For this review, take the finished solid that the model builds, in its own axes (mm). Give positions to 0.01 mm unless a question says otherwise; leave off trailing zeros. Loops run counter-clockwise (first coordinate to the right, second up) from the corner with the lowest first, then second, coordinate; pieces in that order, holes last. Notation, with made-up numbers: (79.25, -21.75) -> (120.25, -21.75) arc R16 cw to (120.25, -15.75) -> close; hole circle Ø5 at (-39.5, 83). An arc over 180 degrees is marked (long way). Write each question's results on one line, items separated by ' | '. Start each with the question number.
```python
from build123d import *

# Parameters (mm, degrees)
SKETCH1_R           = 12.7
BOSS_EXTRUDE1_DEPTH = 58.7248
CHAMFER3_SIZE       = 6.35
CHAMFER3_SIZE2      = 23.698522628
CHAMFER4_SIZE       = 6.35
CHAMFER4_SIZE2      = 23.698522628


with BuildPart() as part:
    # Sketch1 → Boss-Extrude1 (new body)
    with BuildSketch(Plane.XY):
        Circle(SKETCH1_R)
    extrude(amount=-BOSS_EXTRUDE1_DEPTH)

    # Chamfer3
    chamfer3_edges = [part.edges().sort_by_distance(p)[0] for p in [
        (-12.7, 0, -58.7248),
    ]]
    chamfer3_side = [part.faces().sort_by_distance(p)[0] for p in [
        (0, 0, -58.7248),
    ]]
    chamfer(chamfer3_edges, length=CHAMFER3_SIZE, length2=CHAMFER3_SIZE2, reference=chamfer3_side[0])

    # Chamfer4
    chamfer4_edges = [part.edges().sort_by_distance(p)[0] for p in [
        (-12.7, 0, 0),
    ]]
    chamfer4_side = [part.faces().sort_by_distance(p)[0] for p in [
        (0, 0, 0),
    ]]
    chamfer(chamfer4_edges, length=CHAMFER4_SIZE, length2=CHAMFER4_SIZE2, reference=chamfer4_side[0])


solid = part.part
```
1. Wall thickness on L1, parallel to Y at x = 5.75, z = -13; L2, parallel to Y at x = 7.5, z = -36.5; L3, parallel to X at y = -8.75, z = -17: over which ranges is each line inside the solid? List them lowest first.
2. We need section A-A (x = 0). Write out the cut boundary in (y, z).
3. We need section C-C (z = -55). Write out the cut boundary in (x, y).
4. For pin 1 Ø2 at (y, z) = (-2.5, -39) entering from +X; pin 2 Ø2 at (y, z) = (-8, -31) entering from +X; pin 3 Ø8 at (x, z) = (8.5, -27.5) entering from +Y; pin 4 Ø5 at (x, z) = (-1, -22) entering from -Y, all flat-tipped, find the tip position at first contact; note any pin that passes through.
5. We need section D-D (z = -21.5). Write out the cut boundary in (x, y).
Response:
1) L1: y = -7.98 to 7.98 | L2: y = -9.76 to 9.76 | L3: x = -6.51 to 6.51
2) outline: (-12.7, -35.03) -> (-6.35, -58.72) -> (6.35, -58.72) -> (12.7, -35.03) -> (12.7, -23.7) -> (6.35, 0) -> (-6.35, 0) -> (-12.7, -23.7) -> close
3) outline: circle Ø14.7 at (0, 0)
4) pin 1: stops at x = 11.7 | pin 2: stops at x = 10.6 | pin 3: stops at y = 11.88 | pin 4: stops at y = -12.7
5) outline: circle Ø24.22 at (0, 0)
